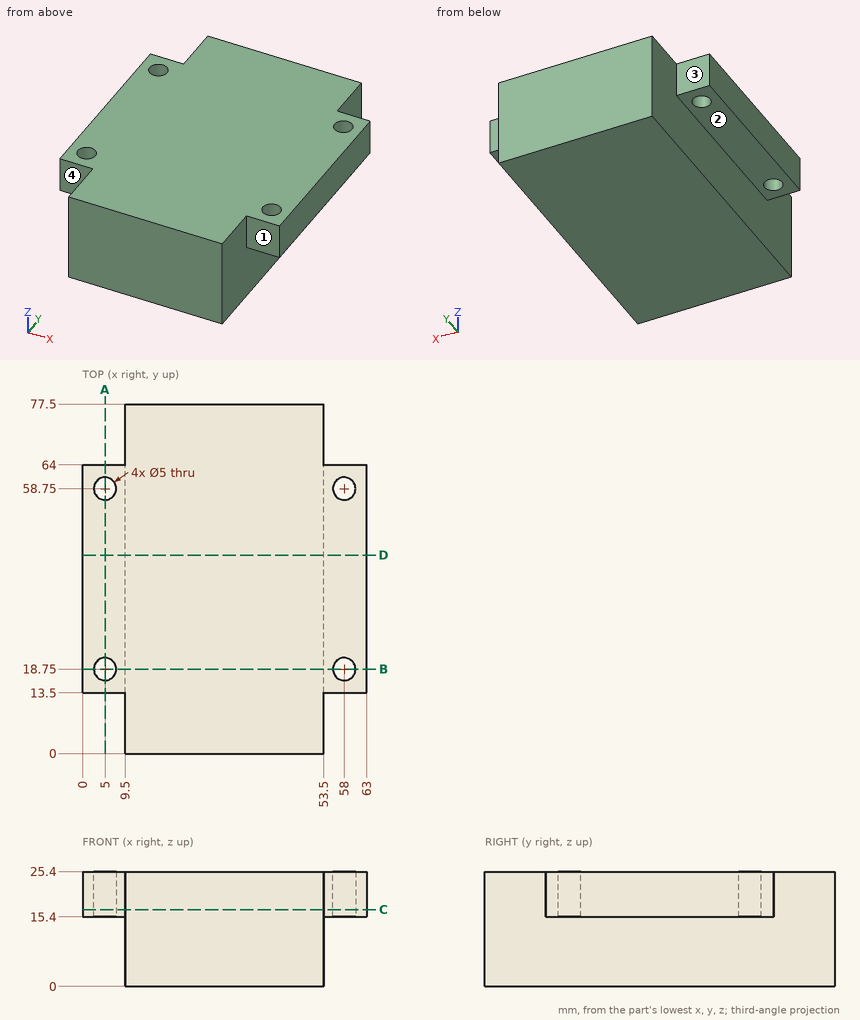
Source: three-view drawing plus pictorial views. Frame: mm from the lowest corner of the part. A direction names the side the tool comes from. Give positions to 0.01 mm unless a question says otherwise; leave off trailing zeros. Loops run counter-clockwise (first coordinate to the right, second up) from the corner with the lowest first, then second, coordinate; pieces in that order, holes last. Notation, with made-up numbers: M 45.5,-31.75 L 51.5,-31.75 A20 ccw 51.5,-9.75 Z; hole C -7.5,83.25 d3. An arc over 180 degrees is marked long. Put each result on its own line as item: value.
Q1. Section D-D (y = 44). Return the cut outline in (x, z).
Response values:
outline: M 0,15.4 L 9.5,15.4 L 9.5,0 L 53.5,0 L 53.5,15.4 L 63,15.4 L 63,25.4 L 0,25.4 Z
Q2. Pin query (flat end, axial travel): P1, Ø5, axis at x = 5.5, y = 41.5, coming from the -Z side; P2, Ø1.5, axis at y = 51, z = 9.5, coming from the +X side; P3, Ø4.5, axis at x = 58, y = 18.75, coming from the +Z side. Return the tip coordinate at first contact, or that it passes through.
Response values:
P1: stops at z = 15.4
P2: stops at x = 53.5
P3: passes through
Q3. Section C-C (z = 17). Return the cut outline in (x, y).
Response values:
outline: M 0,13.5 L 9.5,13.5 L 9.5,0 L 53.5,0 L 53.5,13.5 L 63,13.5 L 63,64 L 53.5,64 L 53.5,77.5 L 9.5,77.5 L 9.5,64 L 0,64 Z; hole C 5,18.75 d5; hole C 5,58.75 d5; hole C 58,18.75 d5; hole C 58,58.75 d5
Q4. Line query: probe 1 along Y at (x, z) = (58, 23); probe 2 along X at (y, z) = (19.5, 19.25); probe 3 along X at (y, z) = (11, 4.25). Output: solid intervals per line, ascending. Write a range as [from, to].
Response values:
probe 1: y = [13.5, 16.25], [21.25, 56.25], [61.25, 64]
probe 2: x = [0, 2.62], [7.38, 55.62], [60.38, 63]
probe 3: x = [9.5, 53.5]
Q5. Reachability of the marked faces 1, 2, 3 and 4 from +Z, -Z, +X, -X, +Y, -Y: full face, straight path, thin tool, end or side. Return the list, or none.
Response values:
face 1: +Z, -Z, +X, -Y
face 2: -Z, -X, +Y, -Y
face 3: +Z, -Z, -X, +Y
face 4: +Z, -Z, -X, -Y
Q6. Section B-B (y = 18.75). Return the cut outline in (x, z).
Response values:
outline: M 0,15.4 L 2.5,15.4 L 2.5,25.4 L 0,25.4 Z; M 7.5,15.4 L 9.5,15.4 L 9.5,0 L 53.5,0 L 53.5,15.4 L 55.5,15.4 L 55.5,25.4 L 7.5,25.4 Z; M 60.5,15.4 L 63,15.4 L 63,25.4 L 60.5,25.4 Z
Q7. Section A-A (x = 5). Return the cut outline in (y, z).
Response values:
outline: M 13.5,15.4 L 16.25,15.4 L 16.25,25.4 L 13.5,25.4 Z; M 21.25,15.4 L 56.25,15.4 L 56.25,25.4 L 21.25,25.4 Z; M 61.25,15.4 L 64,15.4 L 64,25.4 L 61.25,25.4 Z
